Build history of the part. All positions in model axes, mm. Give positions to 0.01 mm unless a question says otherwise; leave off trailing zeros. Order: outer loops, then holes, each group sorted by start corner. A loop starts at its lowest first (then second) coordinate and runs counter-clockwise, first axis right, second up. Notation, with made-up numbers: (89, 48.5) - (119, 48.5) arc R17 ccw to (119, 68.5) - close; hole circle Ø11 at (68, 25). An arc over 180 degrees is marked (long way). Write each question's results on one line, items separated by ' | '. Start each with the question number.
1) Cut at D-D on x = -17. List the corners of the cut face in (y, z), plus the area to 3 significant figures.
2) Drop a flat-ended pin along its axis: pin 1 Ø2.5 at (x, y) = (-17.186, 0) entering from +Z (1 decimal). Give the stop position or say it passes through.
3) Cut at A-A on y = 0. List the corners of the cut face in (x, z), plus the area to 3 significant figures.
4) Cut at B-B on z = 0.5. List the corners of the cut face in (x, y).
5) Cut at C-C on x = 16. List the corners of the cut face in (y, z), plus the area to 3 significant figures.
6) Drill centre lines: line 1 along X through (y, z) = (-7.25, 1.15); line 2 along X through (y, z) = (0.5, 2.45); line 3 along X through (y, z) = (8, 2.1). Where is each one in solid material? Low to high. Write a range as from..to.
from build123d import *

# Parameters (mm, degrees)
SKETCH_W  = 45
SKETCH_H  = 20
SKETCH_R  = 1.6
PAD_DEPTH = 3
FILLET_R  = 3


with BuildPart() as part:
    # Sketch → Pad (new body)
    with BuildSketch(Plane.XY):
        Rectangle(SKETCH_W, SKETCH_H)
        with Locations((-17.186, 0)):
            Circle(SKETCH_R, mode=Mode.SUBTRACT)
        with Locations((17.186, 0)):
            Circle(SKETCH_R, mode=Mode.SUBTRACT)
    extrude(amount=PAD_DEPTH)

    # Fillet
    fillet_edges = [part.edges().sort_by_distance(p)[0] for p in [
        (22.5, 10, 1.5),
        (22.5, -10, 1.5),
        (-22.5, -10, 1.5),
        (-22.5, 10, 1.5),
    ]]
    fillet(fillet_edges, radius=FILLET_R)


solid = part.part
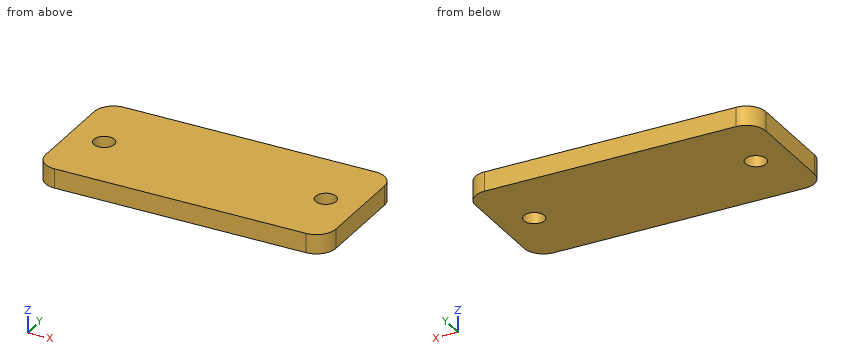
Results:
1) outline: (-10, 0) - (-1.59, 0) - (-1.59, 3) - (-10, 3) - close; (1.59, 0) - (10, 0) - (10, 3) - (1.59, 3) - close | area: 50.5 mm^2
2) pin 1: through
3) outline: (-22.5, 0) - (-18.79, 0) - (-18.79, 3) - (-22.5, 3) - close; (-15.59, 0) - (15.59, 0) - (15.59, 3) - (-15.59, 3) - close; (18.79, 0) - (22.5, 0) - (22.5, 3) - (18.79, 3) - close | area: 116 mm^2
4) outline: (-22.5, -7) arc R3 ccw to (-19.5, -10) - (19.5, -10) arc R3 ccw to (22.5, -7) - (22.5, 7) arc R3 ccw to (19.5, 10) - (-19.5, 10) arc R3 ccw to (-22.5, 7) - close; hole circle Ø3.2 at (-17.19, 0); hole circle Ø3.2 at (17.19, 0)
5) outline: (-10, 0) - (-1.07, 0) - (-1.07, 3) - (-10, 3) - close; (1.07, 0) - (10, 0) - (10, 3) - (1.07, 3) - close | area: 53.6 mm^2
6) line 1: -22.49..22.49 | line 2: -22.5..-18.71, -15.67..15.67, 18.71..22.5 | line 3: -22.33..22.33
